Work out the finished part from the listing and answer in its coordinate system (mm). Face numbers are marked on the shaded views. A direction names the side the tool comes from. Round coordinates to 2 decimals unless told otherwise and drop trailing zeros. Write each loop counter-clockwise with the first axis right and the second up, starting at its lowest first coordinate (ties: lowest second). Pieces come first, ordered by that corner, then holes.
1. Find section B-B (x = 158). Write down the section's boundary in (y, z), and give its area (3 significant figures).
2. Find section C-C (y = 102.5). Write down the section's boundary in (x, z).
3. Determine the mould class of the marked faces 1, 2, 3 and 4 for opening direction Y: pulls with the +Y half, pulls with the -Y half, needs draft (parallel to the pull), parting line crosses it, or undercut.
4. A tool of negligible diameter and unlimited length cuts with its end or side. For the marked faces 5 and 6, from which of +Z, -Z, +X, -X, +Y, -Y can it reach the whole face along a straight path? Write none if from no direction.
5. Straight lines are drawn through the part: probe 1 along Y at (x, z) = (125, 288); probe 2 along X at (y, z) = (99, 156.5); probe 3 along X at (y, z) = (74, 175.5). For each, find the intervals that lie inside material, in ascending order.
6. Flat-ended cylindrical pins translate along their axes: pin 1 Ø1.5 at (y, z) = (50, 113) entering from +X; pin 2 Ø5 at (y, z) = (101.5, 164) entering from +X; pin 3 Ø7 at (x, y) = (200, 96.5) entering from -Z; pin 4 Ø8.5 at (x, y) = (70.5, 27.5) entering from -Z. Find the tip coordinate at first contact, or state that the pin passes through.
7. Find section A-A (z = 138). Write down the section's boundary in (x, y).
8. Find section D-D (z = 286). Write down the section's boundary in (x, y) (3 decimals).
Autodesk Inventor part; units mm, degrees
ref_plane "YZ Plane" through (0, 0, 0) normal (1, 0, 0) x (0, 1, 0)
ref_plane "XZ Plane" through (0, 0, 0) normal (0, 1, 0) x (-1, 0, 0)
ref_plane "XY Plane" through (0, 0, 0) normal (0, 0, 1) x (1, 0, 0)
sketch "Sketch1" plane through (0, 0, 0) normal (0, 0, 1) x (1, 0, 0)
  line L0 (262.89, 151.7796) -> (525.78, 0) construction
  line L1 (525.78, 0) -> (525.78, -303.5592) construction
  line L2 (525.78, -303.5592) -> (262.89, -455.3388) construction
  line L3 (262.89, -455.3388) -> (0, -303.5592) construction
  line L4 (0, -303.5592) -> (0, 0) construction
  line L5 (0, 0) -> (262.89, 151.7796)
  line L6 (0, 0) -> (25.4, -14.6647)
  line L7 (25.4, -14.6647) -> (262.89, 122.4502)
  line L8 (262.89, 122.4502) -> (262.89, 151.7796)
  point P0 (262.89, -151.7796)
  dimension "d0" = 525.78
  dimension "d2" = 25.4
  dimension "d3" = 60
  dimension "d4" = 60
extrude "Extrusion1" add sketch "Sketch1" along normal blind 330.2
sketch "Sketch8" plane through (0, 0, 0) normal (0, 0, -1) x (-1, 0, 0)
  line L0 (-25.4, -14.6647) -> (-262.89, 122.4502)
  line L1 (-198.618, 85.3428) -> (-192.268, 96.3413)
  line L2 (-192.268, 96.3413) -> (-214.265, 109.0413)
  line L3 (-214.265, 109.0413) -> (-220.615, 98.0428)
  line L4 (-198.618, 85.3428) -> (-220.615, 98.0428)
  point P0 (0, 0)
  dimension "d47" = 25.4
  dimension "d48" = 12.7
  dimension "d49" = 48.8149
extrude "Extrusion7" cut sketch "Sketch8" against normal blind 25.4
sketch "Sketch9" plane through (0, 0, 330.2) normal (0, 0, 1) x (1, 0, 0)
  line L0 (192.268, 96.3413) -> (198.618, 85.3428)
  line L1 (214.265, 109.0413) -> (192.268, 96.3413)
  line L2 (220.615, 98.0428) -> (214.265, 109.0413)
  line L3 (198.618, 85.3428) -> (220.615, 98.0428)
  point P0 (0, 0)
extrude "Extrusion8" cut sketch "Sketch9" against normal blind 185
sketch "Sketch10" plane through (25.4, -14.6647, 0) normal (0.5, -0.8660254, 0) x (0.8660254, 0.5, 0)
  line L0 (25.4, 157.9) -> (248.8298, 157.9) construction
  line L1 (248.8298, 157.9) -> (248.8298, 12.7) construction
  line L2 (248.8298, 12.7) -> (25.4, 12.7) construction
  line L3 (25.4, 12.7) -> (25.4, 157.9) construction
  line L4 (225.4149, 145.2) -> (200.0149, 145.2) construction
  line L5 (200.0149, 25.4) -> (225.4149, 25.4) construction
  line L6 (274.2298, 0) -> (274.2298, 330.2) construction
  line L7 (0, 0) -> (0, 330.2) construction
  circle A0 centre (25.4, 157.9) radius 2
  circle A1 centre (25.4, 12.7) radius 2
  circle A2 centre (248.8298, 157.9) radius 2
  circle A3 centre (248.8298, 12.7) radius 2
  point P0 (-14.6647, 0)
  dimension "d54" = 12.7
  dimension "d55" = 12.7
  dimension "d56" = 25.4
  dimension "d57" = 25.4
  dimension "d58" = 4
  dimension "d59" = 4
  dimension "d60" = 4
  dimension "d61" = 4
extrude "Extrusion9" cut sketch "Sketch10" against normal through all
sketch "Sketch11" plane through (0, 0, 330.2) normal (-0.5, 0.8660254, 0) x (0.8660254, 0.5, 0)
  circle A0 centre (263.4945, 172.3) radius 2
  circle A1 centre (263.4945, 317.5) radius 2
  circle A2 centre (40.0647, 317.5) radius 2
  circle A3 centre (40.0647, 172.3) radius 2
  circle A4 centre (263.4945, 172.3) radius 6.5
  circle A5 centre (40.0647, 172.3) radius 2
  circle A6 centre (40.0647, 172.3) radius 6.5
  circle A7 centre (40.0647, 317.5) radius 6.5
  circle A8 centre (263.4945, 317.5) radius 2
  circle A9 centre (263.4945, 317.5) radius 6.5
  point P0 (0, 330.2)
  dimension "d64" = 13
  dimension "d65" = 13
  dimension "d66" = 13
  dimension "d67" = 13
extrude "Extrusion10" cut sketch "Sketch11" against normal blind 12.7 contours A0 | A1 | A2 | A3 | A4 | A6 | A7 | A9
sketch "Sketch12" plane through (0, 0, 330.2) normal (-0.5, 0.8660254, 0) x (0.8660254, 0.5, 0)
  circle A0 centre (115.0647, 269.9) radius 4
  circle A1 centre (115.0647, 219.9) radius 4
  circle A2 centre (40.0647, 317.5) radius 6.5 construction
  circle A3 centre (40.0647, 172.3) radius 6.5 construction
  circle A4 centre (40.0647, 317.5) radius 2
  circle A5 centre (40.0647, 172.3) radius 2
  line L0 (40.0647, 317.5) -> (40.0647, 172.3) construction
  line L1 (115.0647, 269.9) -> (115.0647, 219.9) construction
  point P0 (0, 330.2)
  point P1 (40.0647, 244.9)
  point P2 (115.0647, 244.9)
  dimension "d70" = 8
  dimension "d71" = 8
  dimension "d72" = 75
  dimension "d73" = 50
extrude "Extrusion11" cut sketch "Sketch12" against normal through all contours A0 | A1
sketch "Sketch13" plane through (0, 0, 330.2) normal (-0.5, 0.8660254, 0) x (0.8660254, 0.5, 0)
  circle A0 centre (115.0647, 219.9) radius 4
  circle A1 centre (115.0647, 269.9) radius 4
  circle A2 centre (115.0647, 219.9) radius 7.5
  circle A3 centre (115.0647, 269.9) radius 7.5
  point P0 (0, 330.2)
  dimension "d76" = 15
  dimension "d77" = 15
extrude "Extrusion12" cut sketch "Sketch13" against normal blind 12.7 contours A0 | A1 | A2 | A3
sketch "Sketch14" plane through (25.4, -14.6647, 0) normal (0.5, -0.8660254, 0) x (0.8660254, 0.5, 0)
  line L0 (50.8, 304.8) -> (75, 304.8)
  line L1 (75, 304.8) -> (75, 25.4)
  line L2 (75, 25.4) -> (50.8, 25.4)
  line L3 (50.8, 25.4) -> (50.8, 304.8)
  line L4 (125.8, 25.4) -> (174.6149, 25.4)
  line L5 (174.6149, 25.4) -> (174.6149, 304.8)
  line L6 (174.6149, 304.8) -> (125.8, 304.8)
  line L7 (125.8, 304.8) -> (125.8, 25.4)
  line L8 (174.6149, 119.8) -> (248.8298, 119.8)
  line L9 (248.8298, 119.8) -> (248.8298, 50.8)
  line L10 (248.8298, 50.8) -> (174.6149, 50.8)
  line L11 (174.6149, 50.8) -> (174.6149, 119.8)
  line L12 (0, 330.2) -> (200.0149, 330.2)
  line L13 (0, 0) -> (200.0149, 0)
  line L14 (200.0149, 0) -> (200.0149, 25.4)
  circle A0 centre (100.4, 110.3) radius 4
  circle A1 centre (25.4, 157.9) radius 2
  line L15 (225.4149, 145.2) -> (200.0149, 145.2)
  line L16 (200.0149, 25.4) -> (225.4149, 25.4)
  line L17 (274.2298, 0) -> (274.2298, 330.2)
  point P0 (-14.6647, 0)
  dimension "d80" = 25.4
  dimension "d81" = 25.4
  dimension "d82" = 25.4
  dimension "d83" = 25.4
  dimension "d84" = 25.4
  dimension "d85" = 25.4
  dimension "d86" = 25.4
  dimension "d87" = 25.4
  dimension "d88" = 25.4
extrude "Extrusion13" cut sketch "Sketch14" against normal blind 19.05 contours L0 L1 L2 L3 | L7 L6 L5 L4 | L5 L8 L9 L10
sketch "Sketch15" plane through (0, 0, 330.2) normal (0, 0, 1) x (1, 0, 0)
  line L0 (12.7, -7.3323) -> (262.89, 137.1149) construction
  line L1 (0, 0) -> (25.4, -14.6647)
  line L2 (262.89, 122.4502) -> (262.89, 151.7796)
  line L3 (51.1925, 14.8913) -> (224.3975, 114.8913)
  circle A0 centre (51.1925, 14.8913) radius 2
  circle A1 centre (224.3975, 114.8913) radius 2
  point P0 (137.795, 64.8913)
  dimension "d91" = 200
  dimension "d92" = 4
  dimension "d93" = 4
extrude "Extrusion14" cut sketch "Sketch15" against normal blind 38.1
properties part number "HB02" material "Polyethylene, High Density"
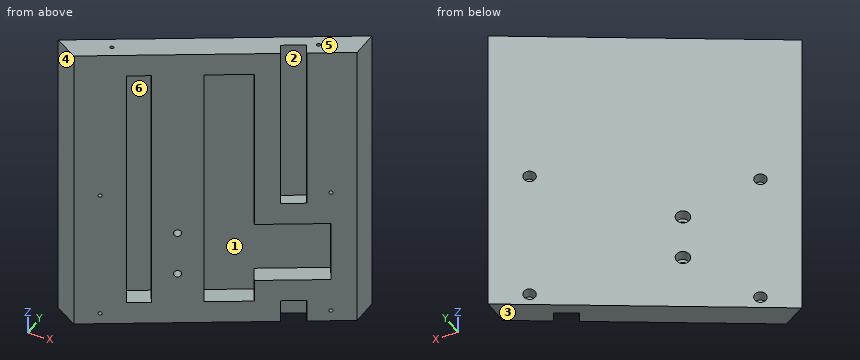
Worked answers:
1. outline: (61.89, 0) - (91.22, 0) - (91.22, 330.2) - (61.89, 330.2) - (61.89, 304.8) - (83.89, 304.8) - (83.89, 25.4) - (61.89, 25.4) - close
1. area: 3,540 mm2
2. outline: (177.54, 0) - (202.94, 0) - (202.94, 25.4) - (218.04, 25.4) - (218.04, 0) - (228.34, 0) - (228.34, 50.8) - (190.23, 50.8) - (190.23, 119.8) - (228.34, 119.8) - (228.34, 330.2) - (218.04, 330.2) - (218.04, 145.2) - (202.94, 145.2) - (202.94, 330.2) - (177.54, 330.2) - close
3. face 1: undercut
3. face 2: undercut
3. face 3: needs draft
3. face 4: pulls with the -Y half
4. face 5: +Z, +X, -X, +Y, -Y
4. face 6: none
5. probe 1: y = 42.84 to 64.42, 64.84 to 72.17
5. probe 2: x = 171.47 to 196.87, 220.06 to 222.27
5. probe 3: x = 128.17 to 140.87, 175.84 to 178.97
6. pin 1: stops at x = 133.76
6. pin 2: stops at x = 230.93
6. pin 3: stops at z = 25.4
6. pin 4: stops at z = 0
7. outline: (0, 0) - (25.4, -14.66) - (69.39, 10.74) - (59.87, 27.23) - (80.83, 39.33) - (90.35, 22.84) - (134.35, 48.24) - (124.82, 64.73) - (167.09, 89.14) - (176.62, 72.64) - (262.89, 122.45) - (262.89, 151.78) - close
8. outline: (0, 0) - (25.4, -14.665) - (69.394, 10.735) - (59.868, 27.235) - (80.826, 39.335) - (90.352, 22.835) - (134.346, 48.235) - (124.82, 64.735) - (167.095, 89.142) - (176.621, 72.643) - (198.618, 85.343) - (192.268, 96.341) - (214.265, 109.041) - (220.615, 98.043) - (262.89, 122.45) - (262.89, 151.78) - close
